Work out the finished part from the listing and answer in its coordinate system (mm). A direction names the side the tool comes from. Round coordinates to 2 decimals unless told otherwise and drop trailing zeros. Loops run counter-clockwise (first coordinate to the right, second up) from the corner with the lowest first, then second, coordinate; pieces in that order, holes last.
```python
from build123d import *

# Parameters (mm, degrees)
SKETCH1_R           = 4
BOSS_EXTRUDE1_DEPTH = 1
BOSS_EXTRUDE2_DEPTH = 3.5
FILLET1_R           = 0.5
FILLET3_R           = 0.5


with BuildPart() as part:
    # Sketch1 → Boss-Extrude1 (new body)
    with BuildSketch(Plane.XY):
        with Locations((-133.270827388, 0)):
            Circle(SKETCH1_R)
    extrude(amount=BOSS_EXTRUDE1_DEPTH)

    # Sketch2 → Boss-Extrude2 (add)
    with BuildSketch(Plane.XY.offset(1)):
        with BuildLine():
            ThreePointArc((-125.3812469, 3.783783784), (-124.520827388, 0), (-125.3812469, -3.783783784))
            ThreePointArc((-125.3812469, -3.783783784), (-142.020827388, 0), (-125.3812469, 3.783783784))
        make_face()
    extrude(amount=BOSS_EXTRUDE2_DEPTH)

    # Fillet1
    fillet1_edges = [part.edges().sort_by_distance(p)[0] for p in [
        (-137.270827388, 0, 1),
        (-141.160407876, -3.783783784, 1),
    ]]
    fillet(fillet1_edges, radius=FILLET1_R)

    # Fillet3
    fillet3_edges = [part.edges().sort_by_distance(p)[0] for p in [
        (-141.160407876, -3.783783784, 4.5),
    ]]
    fillet(fillet3_edges, radius=FILLET3_R)


solid = part.part
```
1. Which of the six approach directions +Z, -Z, +X, -X, +Y, -Y give full straight-line access (tool end or side, diameter ignored) to faces 1 (the face through (-129.456, 1.201, 0.246)), 2 (the face through (-133, 0, 4.5))?
Answer key:
face 1: -Z
face 2: +Z, +X, -X, +Y, -Y
2. Find section A-A (y = 0). Write down the section's boundary in (x, z), then the cut area to 3 significant figures.
Answer key:
outline: (-142.02, 1.5) arc R0.5 ccw to (-141.52, 1) - (-137.77, 1) arc R0.5 cw to (-137.27, 0.5) - (-137.27, 0) - (-129.27, 0) - (-129.27, 0.5) arc R0.5 cw to (-128.77, 1) - (-125.02, 1) arc R0.5 ccw to (-124.52, 1.5) - (-124.52, 4) arc R0.5 ccw to (-125.02, 4.5) - (-141.52, 4.5) arc R0.5 ccw to (-142.02, 4) - close
area: 69.1 mm2
3. Consider probe 1 along Y at (x, z) = (-133.5, 3.4); probe 2 along X at (y, z) = (0.25, 3.95); probe 3 along Z at (x, y) = (-134.25, 4.75). Determine where each line is inside the solid, lowest interval first.
Answer key:
probe 1: y = -8.75 to 8.75
probe 2: x = -142.02 to -124.52
probe 3: z = 1 to 4.5
4. Given pin 1 (5 mm diameter, centred on x = -135.5, y = -0.5, fed in from -Z); pin 2 (1 mm diameter, centred on y = -7, z = 1, fed in from +X); pin 3 (1.5 mm diameter, centred on x = -126.5, y = -0.5, fed in from -Z), each flat-ended and moving along its own axis, determine where each tip first touches the part or whether it passes through.
Answer key:
pin 1: stops at z = 0
pin 2: stops at x = -127.59
pin 3: stops at z = 1
5. Find section B-B (z = 3). Write down the section's boundary in (x, y), then the cut area to 3 significant figures.
Answer key:
outline: circle Ø17.5 at (-133.27, 0)
area: 241 mm2
